Input: part model. Units: mm. Frame: model coordinates. Give positions to 0.01 mm unless a question says otherwise; leave off trailing zeros. Write each loop counter-clockwise with the first axis right and the second up, starting at its lowest first coordinate (ties: lowest second). Pieces come first, ordered by that corner, then holes. Notation, with made-up numbers: (-32, 11) -> (-20, 11) arc R16 cw to (-20, 36) -> close; hole circle Ø9 at (12.5, -8.75). An arc over 180 degrees is marked (long way). Answer as a JSON object with one key per item and string values. Group by question number.
from build123d import *

# Parameters (mm, degrees)
F1_DEPTH = 2.9972
F2_W     = 19.05
F2_H     = 1.5875
F2_R     = 11.1125
F3_DEPTH = 2.9982
F5_DEPTH = 2.9972


with BuildPart() as f1:
    # F0 (on Top) → F1 (new body)
    with BuildSketch(Plane.XY):
        Polygon((-24.3800584922, 42.2275), (-48.7601169844, 0), (-24.3800584922, -42.2275), (24.3800584922, -42.2275), (48.7601169844, 0), (24.3800584922, 42.2275), align=None)
    extrude(amount=F1_DEPTH)

    # F2 (on Top) → F3 (cut, through all)
    with BuildSketch(Plane.XY):
        with Locations((0, 41.43375)):
            Rectangle(F2_W, F2_H)
        with BuildLine():
            Line((-17.272, 42.2275), (-17.272, 41.4655))
            ThreePointArc((-17.272, 41.4655), (-15.875, 39.1239792775), (-14.478, 41.4655))
            Line((-14.478, 41.4655), (-14.478, 42.2275))
            Line((-14.478, 42.2275), (-17.272, 42.2275))
        make_face()
        with BuildLine():
            Line((-24.3800584922, 42.2275), (-25.9675584922, 39.477869343))
            ThreePointArc((-25.9675584922, 39.477869343), (-22.7925584922, 39.477869343), (-21.2050584922, 42.2275))
            Line((-21.2050584922, 42.2275), (-24.3800584922, 42.2275))
        make_face()
        Polygon((-31.8075877383, 29.362641971), (-41.3325877383, 12.864858029), (-39.9577724098, 12.071108029), (-30.4327724098, 28.568891971), align=None)
        with BuildLine():
            Line((-48.7601169844, 0), (-47.1726169844, -2.749630657))
            ThreePointArc((-47.1726169844, -2.749630657), (-45.5851169844, 0), (-47.1726169844, 2.749630657))
            Line((-47.1726169844, 2.749630657), (-48.7601169844, 0))
        make_face()
        with BuildLine():
            Line((-45.2060877383, 6.1557592258), (-44.5461763806, 5.7747592258))
            ThreePointArc((-44.5461763806, 5.7747592258), (-41.8198599514, 5.8138363537), (-43.1491763806, 8.194434204))
            Line((-43.1491763806, 8.194434204), (-43.8090877383, 8.575434204))
            Line((-43.8090877383, 8.575434204), (-45.2060877383, 6.1557592258))
        make_face()
        Polygon((-41.3325877383, -12.864858029), (-31.8075877383, -29.362641971), (-30.4327724098, -28.568891971), (-39.9577724098, -12.071108029), align=None)
        with BuildLine():
            Line((-24.3800584922, -42.2275), (-21.2050584922, -42.2275))
            ThreePointArc((-21.2050584922, -42.2275), (-22.7925584922, -39.477869343), (-25.9675584922, -39.477869343))
            Line((-25.9675584922, -39.477869343), (-24.3800584922, -42.2275))
        make_face()
        with BuildLine():
            Line((-27.9340877383, -36.0717407742), (-27.2741763806, -35.6907407742))
            ThreePointArc((-27.2741763806, -35.6907407742), (-25.9448599514, -33.3101429238), (-28.6711763806, -33.271065796))
            Line((-28.6711763806, -33.271065796), (-29.3310877383, -33.652065796))
            Line((-29.3310877383, -33.652065796), (-27.9340877383, -36.0717407742))
        make_face()
        with Locations((0, -41.43375)):
            Rectangle(F2_W, F2_H)
        with BuildLine():
            Line((24.3800584922, -42.2275), (25.9675584922, -39.477869343))
            ThreePointArc((25.9675584922, -39.477869343), (22.7925584922, -39.477869343), (21.2050584922, -42.2275))
            Line((21.2050584922, -42.2275), (24.3800584922, -42.2275))
        make_face()
        with BuildLine():
            Line((17.272, -42.2275), (17.272, -41.4655))
            ThreePointArc((17.272, -41.4655), (15.875, -39.1239792775), (14.478, -41.4655))
            Line((14.478, -41.4655), (14.478, -42.2275))
            Line((14.478, -42.2275), (17.272, -42.2275))
        make_face()
        Polygon((31.8075877383, -29.362641971), (41.3325877383, -12.864858029), (39.9577724098, -12.071108029), (30.4327724098, -28.568891971), align=None)
        with BuildLine():
            Line((48.7601169844, 0), (47.1726169844, 2.749630657))
            ThreePointArc((47.1726169844, 2.749630657), (45.5851169844, 0), (47.1726169844, -2.749630657))
            Line((47.1726169844, -2.749630657), (48.7601169844, 0))
        make_face()
        with BuildLine():
            Line((45.2060877383, -6.1557592258), (44.5461763806, -5.7747592258))
            ThreePointArc((44.5461763806, -5.7747592258), (41.8198599514, -5.8138363537), (43.1491763806, -8.194434204))
            Line((43.1491763806, -8.194434204), (43.8090877383, -8.575434204))
            Line((43.8090877383, -8.575434204), (45.2060877383, -6.1557592258))
        make_face()
        Polygon((41.3325877383, 12.864858029), (31.8075877383, 29.362641971), (30.4327724098, 28.568891971), (39.9577724098, 12.071108029), align=None)
        with BuildLine():
            Line((24.3800584922, 42.2275), (21.2050584922, 42.2275))
            ThreePointArc((21.2050584922, 42.2275), (22.7925584922, 39.477869343), (25.9675584922, 39.477869343))
            Line((25.9675584922, 39.477869343), (24.3800584922, 42.2275))
        make_face()
        with BuildLine():
            Line((27.9340877383, 36.0717407742), (27.2741763806, 35.6907407742))
            ThreePointArc((27.2741763806, 35.6907407742), (25.9448599514, 33.3101429238), (28.6711763806, 33.271065796))
            Line((28.6711763806, 33.271065796), (29.3310877383, 33.652065796))
            Line((29.3310877383, 33.652065796), (27.9340877383, 36.0717407742))
        make_face()
        Circle(F2_R)
    extrude(amount=F3_DEPTH, mode=Mode.SUBTRACT)

    # F4 (on Top) → F5 (join, through all)
    with BuildSketch(Plane.XY):
        with BuildLine():
            Line((17.272, 42.2275), (17.272, 42.9895))
            ThreePointArc((17.272, 42.9895), (15.875, 45.3310207225), (14.478, 42.9895))
            Line((14.478, 42.9895), (14.478, 42.2275))
            Line((14.478, 42.2275), (17.272, 42.2275))
        make_face()
        with BuildLine():
            Line((-29.990999096, 34.033065796), (-29.3310877383, 33.652065796))
            Line((-29.3310877383, 33.652065796), (-27.9340877383, 36.0717407742))
            Line((-27.9340877383, 36.0717407742), (-28.593999096, 36.4527407742))
            ThreePointArc((-28.593999096, 36.4527407742), (-31.3203155252, 36.4136636463), (-29.990999096, 34.033065796))
        make_face()
        with BuildLine():
            Line((-44.468999096, -8.956434204), (-43.8090877383, -8.575434204))
            Line((-43.8090877383, -8.575434204), (-45.2060877383, -6.1557592258))
            Line((-45.2060877383, -6.1557592258), (-45.865999096, -6.5367592258))
            ThreePointArc((-45.865999096, -6.5367592258), (-47.1953155252, -8.9173570762), (-44.468999096, -8.956434204))
        make_face()
        with BuildLine():
            Line((-14.478, -42.9895), (-14.478, -42.2275))
            Line((-14.478, -42.2275), (-17.272, -42.2275))
            Line((-17.272, -42.2275), (-17.272, -42.9895))
            ThreePointArc((-17.272, -42.9895), (-15.875, -45.3310207225), (-14.478, -42.9895))
        make_face()
        with BuildLine():
            Line((29.990999096, -34.033065796), (29.3310877383, -33.652065796))
            Line((29.3310877383, -33.652065796), (27.9340877383, -36.0717407742))
            Line((27.9340877383, -36.0717407742), (28.593999096, -36.4527407742))
            ThreePointArc((28.593999096, -36.4527407742), (31.3203155252, -36.4136636463), (29.990999096, -34.033065796))
        make_face()
        with BuildLine():
            Line((44.468999096, 8.956434204), (43.8090877383, 8.575434204))
            Line((43.8090877383, 8.575434204), (45.2060877383, 6.1557592258))
            Line((45.2060877383, 6.1557592258), (45.865999096, 6.5367592258))
            ThreePointArc((45.865999096, 6.5367592258), (47.1953155252, 8.9173570762), (44.468999096, 8.956434204))
        make_face()
    extrude(amount=F5_DEPTH)


solid = f1.part
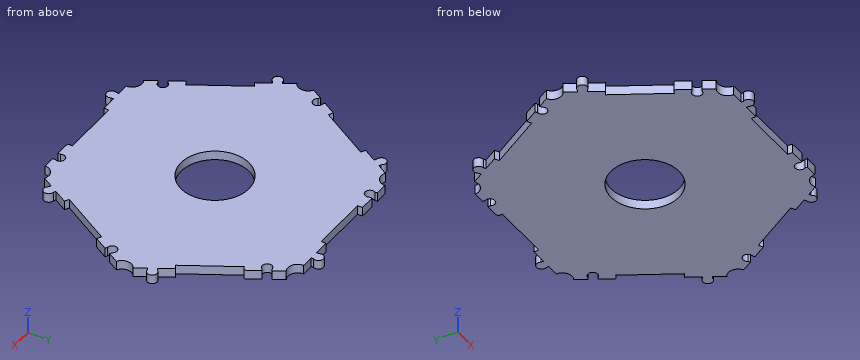
1. Contact query for flat-ended pins moving along their axis: pin 1 Ø1.5 at (x, z) = (-38, 1.5) entering from -Y; pin 2 Ø0.8 at (y, z) = (-42.5, 1.5) entering from -X; pin 3 Ø0.8 at (y, z) = (41, 2) entering from -X. Output: stop coordinate, or through.
2. Line query: line 1 (X direction, y = 42, z = 1.5) (3 decimals); line 2 (X direction, y = 0, z = 1.65); line 3 (X direction, y = -9.5, z = 1.9). Output: solid intervals per line, ascending.
3. Section B-B (x = 0). Return the cut outline in (y, z), plus the area to 3 significant figures.
4. Section A-A (y = 0). Return the cut outline in (x, z), plus the area to 3 significant figures.
5. Section D-D (y = 18). Return the cut outline in (x, z).
6. Section C-C (x = 23). Return the cut outline in (y, z).
Working result:
{
 "1": {"pin 1": "stops at y = -16.76", "pin 2": "stops at x = -21.21", "pin 3": "stops at x = -21.65"},
 "2": {"line 1": "x = -21.213 to -17.272, -14.478 to -9.525, 9.525 to 21.213", "line 2": "x = -45.59 to -11.11, 11.11 to 45.59", "line 3": "x = -46.61 to -45.03, -43.28 to -5.77, 5.77 to 43.28"},
 "3": {"outline": "(-40.64, 0) -> (-11.11, 0) -> (-11.11, 3) -> (-40.64, 3) -> close; (11.11, 0) -> (40.64, 0) -> (40.64, 3) -> (11.11, 3) -> close", "area": "177 mm^2"},
 "4": {"outline": "(-45.59, 0) -> (-11.11, 0) -> (-11.11, 3) -> (-45.59, 3) -> close; (11.11, 0) -> (45.59, 0) -> (45.59, 3) -> (11.11, 3) -> close", "area": "207 mm^2"},
 "5": {"outline": "(-36.53, 0) -> (36.53, 0) -> (36.53, 3) -> (-36.53, 3) -> close"},
 "6": {"outline": "(-39.37, 0) -> (39.37, 0) -> (39.37, 3) -> (-39.37, 3) -> close"}
}
